from build123d import *

# Parameters (mm, degrees)
F4_D    = 25.4
F5_SIZE = 5.08


with BuildPart() as f1:
    # F0 (on Front) → F1 (revolve)
    with BuildSketch(Plane.XZ):
        Polygon((50.8, 0), (-101.6, 0), (-101.6, -38.1), (0, -38.1), (0, -63.5), (50.8, -63.5), align=None)
    revolve(axis=Axis((-25.4, 0, 0), (1, 0, 0)))

    # F4 (through all)
    with Locations(Plane.XZ.offset(38.1)):
        with Locations((-63.5, 0)):
            Hole(F4_D / 2)

    # F5
    f5_edges = [f1.edges().sort_by_distance(p)[0] for p in [
        (50.8, 0, 63.5),
        (-101.6, 0, 38.1),
    ]]
    chamfer(f5_edges, length=F5_SIZE)


solid = f1.part
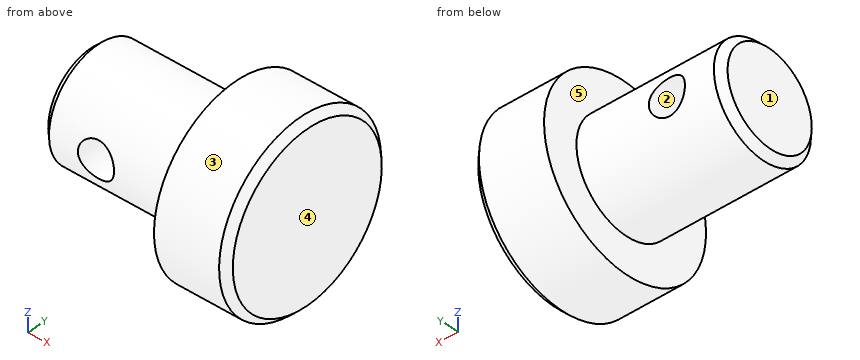
Verification items for the finished model (mm, model axes). Face numbers are marked on the shaded views. A direction names the side the tool comes from. Coordinates: 2 decimals unless noted, no trailing zeros. Loops run counter-clockwise (first coordinate to the right, second up) from the corner with the lowest first, then second, coordinate; pieces in that order, holes last. Notation, with made-up numbers: M 10,3.5 L 21,3.5 A14 cw 21,11.5 Z; hole C -31,65.25 d2. An arc over 180 degrees is marked long. One line per item, written item: value.
1. Section check D-D on x = -63.5. Record the cut outline in (y, z).
Answers follow:
outline: M -35.92,-12.7 A38.1 ccw 35.92,-12.7 Z; M -35.92,12.7 L 35.92,12.7 A38.1 ccw Z
2. Mould release check, pull along Z, two halves, no side actions. Record for the marked faces 1, 2 and 3: pulls with the +Z half, pulls with the -Z half, needs draft (parallel to the pull), parting line crosses it, or undercut.
Answers follow:
face 1: needs draft
face 2: undercut
face 3: parting line crosses it
3. Section check B-B on z = 0. Record the cut outline in (x, y).
Answers follow:
outline: M -101.6,-33.02 L -96.52,-38.1 L -76.2,-38.1 L -76.2,38.1 L -96.52,38.1 L -101.6,33.02 Z; M -50.8,-38.1 L 0,-38.1 L 0,-63.5 L 45.72,-63.5 L 50.8,-58.42 L 50.8,58.42 L 45.72,63.5 L 0,63.5 L 0,38.1 L -50.8,38.1 Z
4. Set-up check for the marked faces 4 and 5: record each of +Z, -Z, +X, -X, +Y, -Y from which the full face is reachable in a straight line by a thin tool's end or side.
Answers follow:
face 4: +Z, -Z, +X, +Y, -Y
face 5: -X
5. Gauge pin test, flat ends, axial feed: P1, Ø4, axis at x = -29.5, y = -10.5, coming from the -Z side; P2, Ø1.5, axis at x = 35, y = 8.5, coming from the +Z side; P3, Ø6, axis at x = 12, z = -5.5, coming from the -Y side. Record the tip position at first contact, or that the pin passes through.
Answers follow:
P1: z = -37.14
P2: z = 63.03
P3: y = -63.45
6. Section check A-A on y = 0. Record the cut outline in (x, z), plus the area to 3 significant figures.
Answers follow:
outline: M -101.6,-33.02 L -96.52,-38.1 L 0,-38.1 L 0,-63.5 L 45.72,-63.5 L 50.8,-58.42 L 50.8,58.42 L 45.72,63.5 L 0,63.5 L 0,38.1 L -96.52,38.1 L -101.6,33.02 Z; hole C -63.5,0 d25.4
area: 13,600 mm^2
7. Material ranges on line 1 along X through (y, z) = (-20.5, 0); line 2 along Z through (x, y) = (-63.5, -8.5); line 3 along X through (y, z) = (-7.5, 11.5), recorded low to high. Write a range as from..to.
Answers follow:
line 1: -101.6..-76.2, -50.8..50.8
line 2: -37.14..-12.7, 12.7..37.14
line 3: -101.6..-68.89, -58.11..50.8
8. Section check C-C on x = 17. Record the cut outline in (y, z), plus the area to 3 significant figures.
Answers follow:
outline: C 0,0 d127
area: 12,700 mm^2
